```python
from build123d import *

# Parameters (mm, degrees)
CHAMFER1_SIZE           = 1
SKETCH2_W               = 3.3
SKETCH2_H               = 3.5
CUT_EXTRUDE1_DEPTH      = 5.725
CUT_EXTRUDE1_DEPTH_BACK = 5.725
SKETCH3_R               = 0.35
CUT_EXTRUDE2_DEPTH      = 5.725
CUT_EXTRUDE2_DEPTH_BACK = 5.725


with BuildPart() as part:
    # Sketch1 → Revolve1 (revolve)
    with BuildSketch(Plane.XY):
        Polygon((-4.725, 0), (-4.725, 7.6), (-3.525, 7.6), (-3.525, 7.3), (-3.225, 7.3), (-3.225, 0), align=None)
    revolve(axis=Axis((0, 7.611752988, 0), (0, -1, 0)))

    # Chamfer1
    chamfer1_edges = [part.edges().sort_by_distance(p)[0] for p in [
        (4.725, 7.6, 0),
    ]]
    chamfer(chamfer1_edges, length=CHAMFER1_SIZE)

    # Sketch2 → Cut-Extrude1 (cut, two sides)
    with BuildSketch(Plane(origin=(0, 0, 0), x_dir=(0, 0, -1), z_dir=(1, 0, 0))) as cut_extrude1_sk:
        with Locations((0, 1.75)):
            Rectangle(SKETCH2_W, SKETCH2_H)
    extrude(amount=CUT_EXTRUDE1_DEPTH, mode=Mode.SUBTRACT)
    extrude(cut_extrude1_sk.sketch, amount=-CUT_EXTRUDE1_DEPTH_BACK, mode=Mode.SUBTRACT)

    # Sketch3 → Cut-Extrude2 (cut, two sides)
    with BuildSketch(Plane.XY) as cut_extrude2_sk:
        with Locations((0, 4.4)):
            Circle(SKETCH3_R)
    extrude(amount=CUT_EXTRUDE2_DEPTH, mode=Mode.SUBTRACT)
    extrude(cut_extrude2_sk.sketch, amount=-CUT_EXTRUDE2_DEPTH_BACK, mode=Mode.SUBTRACT)


solid = part.part
```
Check sheet for the modelled part. Datum: model origin and axes. Units: mm. A direction names the side the tool comes from. Coordinates: 2 decimals unless noted, no trailing zeros. Order: outer loops, then holes, each group sorted by start corner. A loop starts at its lowest first (then second) coordinate and runs counter-clockwise, first axis right, second up. Notation, with made-up numbers: M 4.5,51 L 31.5,51 A11 ccw 31.5,55 Z; hole C 84.25,-14.75 d2. An arc over 180 degrees is marked long. Write each question's results on one line, items separated by ' | '. Start each with the question number.
1. Cross-section at D-D on y = 5. Record the cut outline in (x, z) (3 decimals), and give its area (3 significant figures).
2. Cross-section at A-A on x = 0. Record the cut outline in (y, z) (3 decimals).
3. Cross-section at B-B on z = 0. Record the cut outline in (x, y) (3 decimals).
4. Cross-section at C-C on y = 1.5. Record the cut outline in (x, z) (3 decimals), and give its area (3 significant figures).
5. Access from +Z, -Z, +X, -X, +Y, -Y to the whole of each face (thin tool, end or side, straight path). Record for faces 4 (the face through (4, 3.5, 0)), 5 (the face through (0, 0, -4)), 6 (the face through (2.8, 7.45, 2.14)).
6. Go/stop test with flat-tipped pins: P1, Ø0.6, axis at x = -4, z = -0.5, coming from the -Y side; P2, Ø0.5, axis at x = -3.5, y = 2.5, coming from the -Z side; P3, Ø0.8, axis at x = 4, y = 1.5, coming from the -Z side. Record where each tip stops, or that it passes through.
7. Material ranges on probe 1 along X at (y, z) = (4.4, 3.75); probe 2 along X at (y, z) = (4.4, 4.05); probe 3 along Z at (x, y) = (0, 7.55) (3 decimals), recorded low to high.
8. Mould release check, pull along X, two halves, no side actions. Record for faces 1 (the face through (-4, 3.5, 0)), 2 (the face through (1.024, 3.346, 4.613)), 3 (the face through (3.22, 4.41, -0.14)): +X half, -X half, draft (parallel to the pull), parting line (faces both ways), or undercut.
Checks:
1) outline: C 0,0 d9.45; hole C 0,0 d6.45 | area: 37.5 mm²
2) outline: M 0,-4.725 L 4.05,-4.725 L 4.05,-3.225 L 0,-3.225 Z; M 0,3.225 L 4.05,3.225 L 4.05,4.725 L 0,4.725 Z; M 4.75,-4.725 L 6.6,-4.725 L 7.6,-3.725 L 7.6,-3.525 L 7.3,-3.525 L 7.3,-3.225 L 4.75,-3.225 Z; M 4.75,3.225 L 7.3,3.225 L 7.3,3.525 L 7.6,3.525 L 7.6,3.725 L 6.6,4.725 L 4.75,4.725 Z
3) outline: M -4.725,3.5 L -3.225,3.5 L -3.225,7.3 L -3.525,7.3 L -3.525,7.6 L -3.725,7.6 L -4.725,6.6 Z; M 3.225,3.5 L 4.725,3.5 L 4.725,6.6 L 3.725,7.6 L 3.525,7.6 L 3.525,7.3 L 3.225,7.3 Z
4) outline: M -4.428,-1.65 A4.725 ccw 4.428,-1.65 L 2.771,-1.65 A3.225 cw -2.771,-1.65 Z; M -4.428,1.65 L -2.771,1.65 A3.225 cw 2.771,1.65 L 4.428,1.65 A4.725 ccw Z | area: 27.2 mm²
5) face 4: +X, -X, -Y | face 5: +Z, -Z, +X, -X, -Y | face 6: +Y
6) P1: stops at y = 3.5 | P2: stops at z = -3.43 | P3: stops at z = -3.06
7) probe 1: x = -2.87 to -0.35, 0.35 to 2.87 | probe 2: x = -2.43 to -0.35, 0.35 to 2.43 | probe 3: z = -3.775 to -3.525, 3.525 to 3.775
8) face 1: draft | face 2: parting line | face 3: undercut
